Input: dimensioned drawing with shaded views. Units: mm. Origin: part minimum x, y, z. A direction names the side the tool comes from. Round coordinates to 2 decimals unless told otherwise and drop trailing zeros. Loops run counter-clockwise (first coordinate to the right, second up) from the corner with the lowest first, then second, coordinate; pieces in that order, holes last. Notation, with made-up numbers: M 81,-3 L 100,-3 A9 ccw 100,14 Z; hole C 77.5,-11.5 d9. An arc over 180 degrees is marked long. One line per item, written item: value.
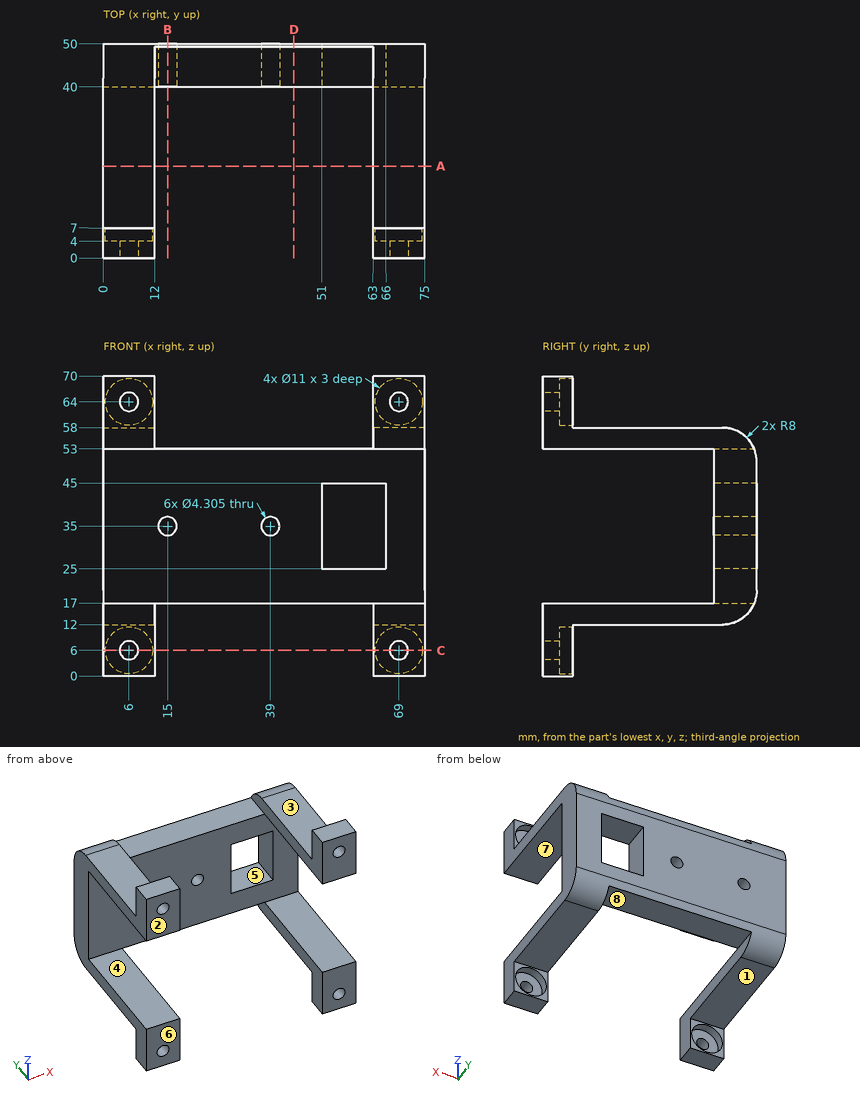
1. Section query A-A (y = 21.5). Return the cut outline in (x, z).
Report:
outline: M 0,12 L 12,12 L 12,17 L 0,17 Z; M 0,53 L 12,53 L 12,58 L 0,58 Z; M 63,12 L 75,12 L 75,17 L 63,17 Z; M 63,53 L 75,53 L 75,58 L 63,58 Z
2. Pull-direction query (Z, two-part tool) for the marked faces 5, 6, 7 and 8; classes: released by +Z, released by -Z, zero draft, split by the parting line, or undercut.
Report:
face 5: undercut
face 6: zero draft
face 7: undercut
face 8: released by -Z
3. Section query B-B (x = 15). Return the cut outline in (y, z).
Report:
outline: M 40,17 L 49.42,17 A8 ccw 50,20 L 50,32.85 L 40,32.85 Z; M 40,37.15 L 50,37.15 L 50,50 A8 ccw 49.42,53 L 40,53 Z
4. Section query D-D (x = 44.5). Return the cut outline in (y, z).
Report:
outline: M 40,17 L 49.42,17 A8 ccw 50,20 L 50,50 A8 ccw 49.42,53 L 40,53 Z
5. Section query C-C (z = 6). Return the cut outline in (x, y).
Report:
outline: M 0,0 L 3.85,0 L 3.85,4 L 0.5,4 L 0.5,7 L 0,7 Z; M 8.15,0 L 12,0 L 12,7 L 11.5,7 L 11.5,4 L 8.15,4 Z; M 63,0 L 66.85,0 L 66.85,4 L 63.5,4 L 63.5,7 L 63,7 Z; M 71.15,0 L 75,0 L 75,7 L 74.5,7 L 74.5,4 L 71.15,4 Z
6. Ray query, line 1 (X direction, y = 6, z = 6); line 2 (X direction, y = 1.15, z = 64); line 3 (Z direction, x = 6, y = 2.7). Return the intervals inside material, ascending. Write a range as [from, to].
Report:
line 1: x = [0, 0.5], [11.5, 12], [63, 63.5], [74.5, 75]
line 2: x = [0, 3.85], [8.15, 12], [63, 66.85], [71.15, 75]
line 3: z = [0, 3.85], [8.15, 17], [53, 61.85], [66.15, 70]
7. Pin query (flat end, axial travel): pin 1 (12 mm diameter, centred on x = 66.5, z = 61.5, fed in from +Y); pin 2 (2 mm diameter, centred on x = 33.5, z = 41, fed in from -Y); pin 3 (10 mm diameter, centred on x = 6, z = 6, fed in from +Y). Return the tip coordinate at first contact, or that it passes through.
Report:
pin 1: stops at y = 47.81
pin 2: stops at y = 40
pin 3: stops at y = 4
8. Reachability of the marked faces 1, 2, 3 and 4 from +Z, -Z, +X, -X, +Y, -Y: full face, straight path, thin tool, end or side. Return the list, or none.
Report:
face 1: -Z, +X, -X, +Y
face 2: +Z, -Z, +X, -X, -Y
face 3: +Z, +X, -X, +Y
face 4: +X, -X, -Y
